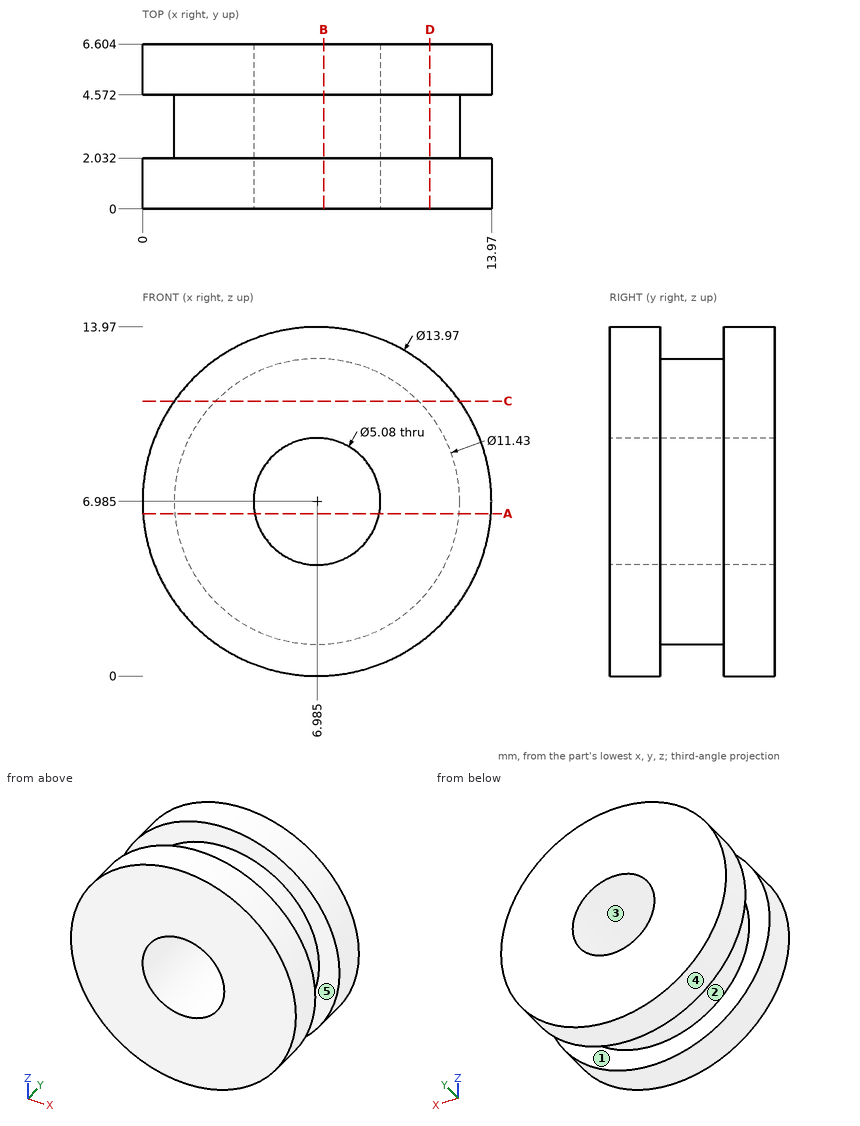
Could you check a few things on this drawing? It's one solid part, dimensions in mm from its lowest x, y, z. A direction names the side the tool comes from. Give positions to 0.01 mm unless a question says otherwise; leave off trailing zeros. Order: outer loops, then holes, each group sorted by start corner. A loop starts at its lowest first (then second) coordinate and runs counter-clockwise, first axis right, second up. Notation, with made-up numbers: (-13, 13.5) -> (6, 13.5) arc R5 ccw to (6, 22.5) -> close; hole circle Ø9 at (10.25, -35.75). An arc over 180 degrees is marked (long way). Answer in a Markdown table with one row per item. Add a question column.
Item 1: Imagine slicing it at D-D (x = 11.5). List the corners of the cut face in (y, z) for me.
Item 2: For the marked faces 4 and 5, which set-ups out of +Z, -Z, +X, -X, +Y, -Y let a thin tool reach every point of the face, with its end or its side?
Item 3: Imagine slicing it at B-B (x = 7.25). List the corners of the cut face in (y, z) for me.
Item 4: I'm going to push a flat-ended pin straight in: P1, Ø1, axis at x = 8, y = 1.5, coming from the -Z side. Where does the tip first touch, or does it pass through?
Item 5: Please list where these lines run through material, in increasing order: probe 1 along Y at (x, z) = (1, 9.5); probe 2 along X at (y, z) = (4.25, 5.5); probe 3 along Z at (x, y) = (8.5, 4).
Item 6: Imagine slicing it at A-A (z = 6.5). List the corners of the cut face in (x, y) for me, and give its area (3 significant figures).
Item 7: Imagine slicing it at C-C (z = 11). List the corners of the cut face in (x, y) for me.
Item 8: We'd pull the mould along Z, two halves only. Please class the marked faces 1, 2 and 3: pulls with the +Z half, pulls with the -Z half, needs draft (parallel to the pull), parting line crosses it, or undercut.
Result:
| question | item | result |
|---|---|---|
| 1 | outline | (0, 1.66) -> (2.03, 1.66) -> (2.03, 3.48) -> (4.57, 3.48) -> (4.57, 1.66) -> (6.6, 1.66) -> (6.6, 12.31) -> (4.57, 12.31) -> (4.57, 10.49) -> (2.03, 10.49) -> (2.03, 12.31) -> (0, 12.31) -> close |
| 2 | face 4 | +Y, -Y |
| 2 | face 5 | none |
| 3 | outline | (0, 0.01) -> (2.03, 0.01) -> (2.03, 1.28) -> (4.57, 1.28) -> (4.57, 0.01) -> (6.6, 0.01) -> (6.6, 4.46) -> (0, 4.46) -> close; (0, 9.51) -> (6.6, 9.51) -> (6.6, 13.96) -> (4.57, 13.96) -> (4.57, 12.69) -> (2.03, 12.69) -> (2.03, 13.96) -> (0, 13.96) -> close |
| 4 | P1 | z = 0.02 |
| 5 | probe 1 | 0 to 2.03, 4.57 to 6.6 |
| 5 | probe 2 | 1.47 to 4.92, 9.05 to 12.5 |
| 5 | probe 3 | 1.47 to 4.95, 9.02 to 12.5 |
| 6 | outline | (0.02, 0) -> (4.49, 0) -> (4.49, 6.6) -> (0.02, 6.6) -> (0.02, 4.57) -> (1.29, 4.57) -> (1.29, 2.03) -> (0.02, 2.03) -> close; (9.48, 0) -> (13.95, 0) -> (13.95, 2.03) -> (12.68, 2.03) -> (12.68, 4.57) -> (13.95, 4.57) -> (13.95, 6.6) -> (9.48, 6.6) -> close |
| 6 | area | 52.6 mm2 |
| 7 | outline | (1.27, 0) -> (12.7, 0) -> (12.7, 2.03) -> (11.05, 2.03) -> (11.05, 4.57) -> (12.7, 4.57) -> (12.7, 6.6) -> (1.27, 6.6) -> (1.27, 4.57) -> (2.92, 4.57) -> (2.92, 2.03) -> (1.27, 2.03) -> close |
| 8 | face 1 | needs draft |
| 8 | face 2 | parting line crosses it |
| 8 | face 3 | undercut |
